CAD build for the part. Positions are in the model's coordinates, mm. A direction names the side the tool comes from. Coordinates: 2 decimals unless noted, no trailing zeros. Loops run counter-clockwise (first coordinate to the right, second up) from the corner with the lowest first, then second, coordinate; pieces in that order, holes last. Notation, with made-up numbers: (22.5, -37) -> (41.5, -37) arc R15 ccw to (41.5, -22) -> close; hole circle Ø8 at (-15.5, 4.5). An arc over 180 degrees is marked (long way). Write each question's results on one line, items separated by ' | '.
from build123d import *

# Parameters (mm, degrees)
SKETCH1_W                                 = 60
SKETCH1_H                                 = 60
BOSS_EXTRUDE1_DEPTH                       = 3
SKETCH2_R                                 = 10.25
CUT_EXTRUDE1_DEPTH                        = 43.532340636
SKETCH4_R                                 = 1.45
STOP_MOUNT_D2P9_THROUGH_DEPTH             = 3.01
SKETCH5_R                                 = 1.45
SERVO_X_MOUNT_D2P9_DEPTH                  = 3.01
SKETCH6_R                                 = 1.2
GUIDERAIL2_D2P4_DEPTH                     = 3.01
SKETCH12_W                                = 15
SKETCH12_H                                = 6
ROUTED_FRAME_EAR_LEFTPLUS_ROOT_DEPTH      = 3
SKETCH13_W                                = 6
SKETCH13_H                                = 46
ROUTED_FRAME_EAR_LEFTPLUS_OUTBOARD_DEPTH  = 3
SKETCH14_W                                = 22
SKETCH14_H                                = 8
ROUTED_FRAME_EAR_LEFTPLUS_PAD_DEPTH       = 3
SKETCH15_W                                = 15
SKETCH15_H                                = 6
ROUTED_FRAME_EAR_LEFTMINUS_ROOT_DEPTH     = 3
SKETCH16_W                                = 6
SKETCH16_H                                = 46
ROUTED_FRAME_EAR_LEFTMINUS_OUTBOARD_DEPTH = 3
SKETCH17_W                                = 22
SKETCH17_H                                = 8
ROUTED_FRAME_EAR_LEFTMINUS_PAD_DEPTH      = 3
SKETCH18_W                                = 6
SKETCH18_H                                = 8
ROUTED_FRAME_EAR_RIGHTPLUS_ROOT_DEPTH     = 3
SKETCH19_W                                = 8
SKETCH19_H                                = 22
ROUTED_FRAME_EAR_RIGHTPLUS_PAD_DEPTH      = 3
SKETCH20_W                                = 6
SKETCH20_H                                = 8
ROUTED_FRAME_EAR_RIGHTMINUS_ROOT_DEPTH    = 3
SKETCH21_W                                = 8
SKETCH21_H                                = 22
ROUTED_FRAME_EAR_RIGHTMINUS_PAD_DEPTH     = 3
SKETCH22_R                                = 1.7
ROUTED_FRAME_EARS_D3P4_DEPTH              = 3.01
SKETCH23_W                                = 6
SKETCH23_H                                = 20
FOUR_LINK_SUPPORT_PLUS_LEFTRAIL_DEPTH     = 3
SKETCH24_W                                = 22
SKETCH24_H                                = 8
FOUR_LINK_SUPPORT_PLUS_LEFTPAD_DEPTH      = 3
SKETCH25_W                                = 8
SKETCH25_H                                = 20
FOUR_LINK_SUPPORT_PLUS_RIGHTRAIL_DEPTH    = 3
SKETCH26_W                                = 6
SKETCH26_H                                = 20
FOUR_LINK_SUPPORT_MINUS_LEFTRAIL_DEPTH    = 3
SKETCH27_W                                = 22
SKETCH27_H                                = 8
FOUR_LINK_SUPPORT_MINUS_LEFTPAD_DEPTH     = 3
SKETCH28_W                                = 8
SKETCH28_H                                = 20
FOUR_LINK_SUPPORT_MINUS_RIGHTRAIL_DEPTH   = 3
SKETCH29_R                                = 1.7
FOUR_LINK_SUPPORT_HOLES_Y70_DEPTH         = 3.01


with BuildPart() as part:
    # Sketch1 → Boss-Extrude1 (new body)
    with BuildSketch(Plane.XY):
        Rectangle(SKETCH1_W, SKETCH1_H)
    extrude(amount=BOSS_EXTRUDE1_DEPTH)

    # Sketch2 → Cut-Extrude1 (cut, through all)
    with BuildSketch(Plane.XY.offset(3)):
        Circle(SKETCH2_R)
    extrude(amount=-CUT_EXTRUDE1_DEPTH, mode=Mode.SUBTRACT)

    # Sketch4 → Stop_Mount_D2p9_Through (cut)
    with BuildSketch(Plane(origin=(0, 0, 0), x_dir=(-1, 0, 0), z_dir=(0, 0, -1))):
        with Locations((-24, 21)):
            Circle(SKETCH4_R)
        with Locations((-27, 27)):
            Circle(SKETCH4_R)
    extrude(amount=-STOP_MOUNT_D2P9_THROUGH_DEPTH, mode=Mode.SUBTRACT)

    # Sketch5 → Servo_X_Mount_D2p9 (cut)
    with BuildSketch(Plane(origin=(0, 0, 0), x_dir=(-1, 0, 0), z_dir=(0, 0, -1))):
        with Locations((25, 18)):
            Circle(SKETCH5_R)
        with Locations((25, 25)):
            Circle(SKETCH5_R)
    extrude(amount=-SERVO_X_MOUNT_D2P9_DEPTH, mode=Mode.SUBTRACT)

    # Sketch6 → GuideRail2_D2p4 (cut)
    with BuildSketch(Plane.XY.offset(3)):
        with Locations((15, -24)):
            Circle(SKETCH6_R)
        with Locations((0, -24)):
            Circle(SKETCH6_R)
        with Locations((-15, -24)):
            Circle(SKETCH6_R)
    extrude(amount=-GUIDERAIL2_D2P4_DEPTH, mode=Mode.SUBTRACT)

    # Sketch12 → Routed_Frame_Ear_LeftPlus_Root (add)
    with BuildSketch(Plane.XY):
        with Locations((-34.5, 13)):
            Rectangle(SKETCH12_W, SKETCH12_H)
    extrude(amount=ROUTED_FRAME_EAR_LEFTPLUS_ROOT_DEPTH)

    # Sketch13 → Routed_Frame_Ear_LeftPlus_Outboard (add)
    with BuildSketch(Plane.XY):
        with Locations((-39, 33)):
            Rectangle(SKETCH13_W, SKETCH13_H)
    extrude(amount=ROUTED_FRAME_EAR_LEFTPLUS_OUTBOARD_DEPTH)

    # Sketch14 → Routed_Frame_Ear_LeftPlus_Pad (add)
    with BuildSketch(Plane.XY):
        with Locations((-31, 52)):
            Rectangle(SKETCH14_W, SKETCH14_H)
    extrude(amount=ROUTED_FRAME_EAR_LEFTPLUS_PAD_DEPTH)

    # Sketch15 → Routed_Frame_Ear_LeftMinus_Root (add)
    with BuildSketch(Plane.XY):
        with Locations((-34.5, -13)):
            Rectangle(SKETCH15_W, SKETCH15_H)
    extrude(amount=ROUTED_FRAME_EAR_LEFTMINUS_ROOT_DEPTH)

    # Sketch16 → Routed_Frame_Ear_LeftMinus_Outboard (add)
    with BuildSketch(Plane.XY):
        with Locations((-39, -33)):
            Rectangle(SKETCH16_W, SKETCH16_H)
    extrude(amount=ROUTED_FRAME_EAR_LEFTMINUS_OUTBOARD_DEPTH)

    # Sketch17 → Routed_Frame_Ear_LeftMinus_Pad (add)
    with BuildSketch(Plane.XY):
        with Locations((-31, -52)):
            Rectangle(SKETCH17_W, SKETCH17_H)
    extrude(amount=ROUTED_FRAME_EAR_LEFTMINUS_PAD_DEPTH)

    # Sketch18 → Routed_Frame_Ear_RightPlus_Root (add)
    with BuildSketch(Plane.XY):
        with Locations((20, 32)):
            Rectangle(SKETCH18_W, SKETCH18_H)
    extrude(amount=ROUTED_FRAME_EAR_RIGHTPLUS_ROOT_DEPTH)

    # Sketch19 → Routed_Frame_Ear_RightPlus_Pad (add)
    with BuildSketch(Plane.XY):
        with Locations((24, 45)):
            Rectangle(SKETCH19_W, SKETCH19_H)
    extrude(amount=ROUTED_FRAME_EAR_RIGHTPLUS_PAD_DEPTH)

    # Sketch20 → Routed_Frame_Ear_RightMinus_Root (add)
    with BuildSketch(Plane.XY):
        with Locations((20, -32)):
            Rectangle(SKETCH20_W, SKETCH20_H)
    extrude(amount=ROUTED_FRAME_EAR_RIGHTMINUS_ROOT_DEPTH)

    # Sketch21 → Routed_Frame_Ear_RightMinus_Pad (add)
    with BuildSketch(Plane.XY):
        with Locations((24, -45)):
            Rectangle(SKETCH21_W, SKETCH21_H)
    extrude(amount=ROUTED_FRAME_EAR_RIGHTMINUS_PAD_DEPTH)

    # Sketch22 → Routed_Frame_Ears_D3p4 (cut)
    with BuildSketch(Plane.XY.offset(3)):
        with Locations((-24, -52)):
            Circle(SKETCH22_R)
        with Locations((-24, 52)):
            Circle(SKETCH22_R)
        with Locations((24, -52)):
            Circle(SKETCH22_R)
        with Locations((24, 52)):
            Circle(SKETCH22_R)
    extrude(amount=-ROUTED_FRAME_EARS_D3P4_DEPTH, mode=Mode.SUBTRACT)

    # Sketch23 → Four_Link_Support_Plus_LeftRail (add)
    with BuildSketch(Plane.XY):
        with Locations((-39, 64)):
            Rectangle(SKETCH23_W, SKETCH23_H)
    extrude(amount=FOUR_LINK_SUPPORT_PLUS_LEFTRAIL_DEPTH)

    # Sketch24 → Four_Link_Support_Plus_LeftPad (add)
    with BuildSketch(Plane.XY):
        with Locations((-31, 70)):
            Rectangle(SKETCH24_W, SKETCH24_H)
    extrude(amount=FOUR_LINK_SUPPORT_PLUS_LEFTPAD_DEPTH)

    # Sketch25 → Four_Link_Support_Plus_RightRail (add)
    with BuildSketch(Plane.XY):
        with Locations((24, 64)):
            Rectangle(SKETCH25_W, SKETCH25_H)
    extrude(amount=FOUR_LINK_SUPPORT_PLUS_RIGHTRAIL_DEPTH)

    # Sketch26 → Four_Link_Support_Minus_LeftRail (add)
    with BuildSketch(Plane.XY):
        with Locations((-39, -64)):
            Rectangle(SKETCH26_W, SKETCH26_H)
    extrude(amount=FOUR_LINK_SUPPORT_MINUS_LEFTRAIL_DEPTH)

    # Sketch27 → Four_Link_Support_Minus_LeftPad (add)
    with BuildSketch(Plane.XY):
        with Locations((-31, -70)):
            Rectangle(SKETCH27_W, SKETCH27_H)
    extrude(amount=FOUR_LINK_SUPPORT_MINUS_LEFTPAD_DEPTH)

    # Sketch28 → Four_Link_Support_Minus_RightRail (add)
    with BuildSketch(Plane.XY):
        with Locations((24, -64)):
            Rectangle(SKETCH28_W, SKETCH28_H)
    extrude(amount=FOUR_LINK_SUPPORT_MINUS_RIGHTRAIL_DEPTH)

    # Sketch29 → Four_Link_Support_Holes_Y70 (cut)
    with BuildSketch(Plane.XY.offset(3)):
        with Locations((-24, -70)):
            Circle(SKETCH29_R)
        with Locations((-24, 70)):
            Circle(SKETCH29_R)
        with Locations((24, -70)):
            Circle(SKETCH29_R)
        with Locations((24, 70)):
            Circle(SKETCH29_R)
    extrude(amount=-FOUR_LINK_SUPPORT_HOLES_Y70_DEPTH, mode=Mode.SUBTRACT)


solid = part.part
1) Two-plate mould, pull along X, no slides. Class faces 1 (the flat face through (20, 55, 1)), 2 (the flat face through (24, 74, 1)), 3 (the flat face through (28, -54, 1)): pulls with the +X half, pulls with the -X half, needs draft (parallel to the pull), parting line crosses it, or undercut.
Outcome:
face 1: undercut | face 2: needs draft | face 3: pulls with the +X half
2) Pin check, flat tips, straight feed: pin 1 (0.9 mm diameter, centred on y = 31, z = 1, fed in from +X); pin 2 (2.5 mm diameter, centred on x = 27, y = 27, fed in from -Z); pin 3 (1.5 mm diameter, centred on y = 45.5, z = 1.5, fed in from +X); pin 4 (0.9 mm diameter, centred on x = 18.5, z = 2, fed in from +Y). Stop position of each tip, or through.
Outcome:
pin 1: stops at x = 23 | pin 2: passes through | pin 3: stops at x = 28 | pin 4: stops at y = 36
3) Slice it at C-C (y = -63.5). Write the cut outline in (x, z).
Outcome:
outline: (-42, 0) -> (-36, 0) -> (-36, 3) -> (-42, 3) -> close; (20, 0) -> (28, 0) -> (28, 3) -> (20, 3) -> close
4) Which spindle directions (+Z, -Z, +X, -X, +Y, -Y) get a long thin tool onto all of the face, cutting with end or side? Do faces 4 (the flat face through (-20, 70, 1)), 5 (the flat face through (17, -33, 1)), 6 (the flat face through (-7, -30, 1)). Say none if no direction does.
Outcome:
face 4: +Z, -Z, +Y | face 5: +Z, -Z, -Y | face 6: +Z, -Z
5) Slice it at B-B (y = 52). Write the cut outline in (x, z).
Outcome:
outline: (-42, 0) -> (-25.7, 0) -> (-25.7, 3) -> (-42, 3) -> close; (-22.3, 0) -> (-20, 0) -> (-20, 3) -> (-22.3, 3) -> close; (20, 0) -> (22.3, 0) -> (22.3, 3) -> (20, 3) -> close; (25.7, 0) -> (28, 0) -> (28, 3) -> (25.7, 3) -> close
6) Drill centre lines: L1, parallel to X at y = 70, z = 1.7; L2, parallel to Y at x = 0, z = 1.4; L3, parallel to Y at x = -34, z = 2.6. Where is each one in solid material? Low to high. Write a range as from..to.
Outcome:
L1: x = -42..-25.7, -22.3..-20, 20..22.3, 25.7..28 | L2: y = -30..-25.2, -22.8..-10.25, 10.25..30 | L3: y = -74..-66, -56..-48, -16..-10, 10..16, 48..56, 66..74
7) Slice it at A-A (y = 21). Write the cut outline in (x, z).
Outcome:
outline: (-42, 0) -> (-36, 0) -> (-36, 3) -> (-42, 3) -> close; (-30, 0) -> (22.55, 0) -> (22.55, 3) -> (-30, 3) -> close; (25.45, 0) -> (30, 0) -> (30, 3) -> (25.45, 3) -> close
8) Slice it at D-D (z = 2.4). Count the separate pieces of the cut face and the enclosed holes in it, then the cut area to 3 significant figures.
Outcome:
separate pieces: 1 | enclosed holes: 16 | area: 5,210 mm^2
